```python
from build123d import *
from build123d.topology import SkipClean

# Parameters (mm, degrees)
ESBO_O1_W                = 2
ESBO_O1_H                = 46
RESSALTO_EXTRUS_O1_DEPTH = 10
ESBO_O2_W                = 46
ESBO_O2_H                = 46
RESSALTO_EXTRUS_O2_DEPTH = 3
ESBO_O1_4_W              = 2
ESBO_O1_4_H              = 46
RESSALTO_EXTRUS_O3_DEPTH = 11
ESBO_O3_R                = 11
CORTE_EXTRUS_O1_DEPTH    = 11


with BuildPart() as part:
    # Esbo_o1 → Ressalto-extrus_o1 (new body)
    with BuildSketch(Plane(origin=(0, 0, 0), x_dir=(1, 0, 0), z_dir=(0, 1, 0))):
        Polygon((0, -23), (0, -21), (-19, -21), (-19, 21), (19, 21), (19, 0), (19, -21), (5, -21), (5, -23), (7, -23), (21, -23), (21, 23), (7, 23), (3.4e-08, 23), (-7, 23), (-21, 23), (-21, -23), (-7, -23), align=None)
        Polygon((5, -21), (0, -21), (0, -23), (4.898979486, -23), (5, -23), align=None)
        with Locations((-22, 0)):
            Rectangle(ESBO_O1_W, ESBO_O1_H)
        with Locations((22, 0)):
            Rectangle(ESBO_O1_W, ESBO_O1_H)
    extrude(amount=RESSALTO_EXTRUS_O1_DEPTH)

    # Esbo_o2 → Ressalto-extrus_o2 (add)
    # profile 1 of 2: a face of its own
    with BuildSketch(Plane(origin=(0, 10, 0), x_dir=(1, 0, 0), z_dir=(0, 1, 0))):
        Rectangle(ESBO_O2_W, ESBO_O2_H)
        Polygon((19, 21), (19, 11), (19, -11), (19, -21), (-19, -21), (-19, 21), align=None, mode=Mode.SUBTRACT)
    # profile 2 of 2: a face of its own
    with BuildSketch(Plane(origin=(0, 10, 0), x_dir=(1, 0, 0), z_dir=(0, 1, 0))):
        Polygon((-9, -11), (-9, 11), (9, 11), (19, 11), (19, 21), (-19, 21), (-19, -21), (19, -21), (19, -11), (9, -11), align=None)
    extrude(amount=RESSALTO_EXTRUS_O2_DEPTH)

    # Esbo_o1_4 → Ressalto-extrus_o3 (add)
    # profile 1 of 6: a face of its own
    with SkipClean():  # the faces are left unmerged after this step: merging them gives an invalid solid
        with BuildSketch(Plane(origin=(0, 0, 0), x_dir=(1, 0, 0), z_dir=(0, 1, 0))):
            Polygon((0, -23), (0, -21), (-19, -21), (-19, 21), (19, 21), (19, 0), (19, -21), (5, -21), (5, -23), (7, -23), (21, -23), (21, 23), (7, 23), (3.4e-08, 23), (-7, 23), (-21, 23), (-21, -23), (-7, -23), align=None)
        # profile 2 of 6: a face of its own
        with BuildSketch(Plane(origin=(0, 0, 0), x_dir=(1, 0, 0), z_dir=(0, 1, 0))):
            with BuildLine():
                Line((4.898979486, -23), (0, -23))
                Line((0, -23), (-7, -23))
                Line((-7, -23), (-7, -28))
                ThreePointArc((-7, -28), (0, -35), (7, -28))
                Line((7, -28), (7, -23))
                Line((7, -23), (5, -23))
                Line((5, -23), (5, -23.101020514))
                ThreePointArc((5, -23.101020514), (4.949747468, -23.050252532), (4.898979486, -23))
            make_face()
            with BuildLine():
                ThreePointArc((5, -28), (-3.535533906, -31.535533906), (0, -23))
                ThreePointArc((0, -23), (3.535533906, -24.464466094), (5, -28))
            make_face(mode=Mode.SUBTRACT)
        # profile 3 of 6: a face of its own
        with BuildSketch(Plane(origin=(0, 0, 0), x_dir=(1, 0, 0), z_dir=(0, 1, 0))):
            Polygon((5, -21), (0, -21), (0, -23), (4.898979486, -23), (5, -23), align=None)
        # profile 4 of 6: a face of its own
        with BuildSketch(Plane(origin=(0, 0, 0), x_dir=(1, 0, 0), z_dir=(0, 1, 0))):
            with Locations((22, 0)):
                Rectangle(ESBO_O1_4_W, ESBO_O1_4_H)
        # profile 5 of 6: a face of its own
        with BuildSketch(Plane(origin=(0, 0, 0), x_dir=(1, 0, 0), z_dir=(0, 1, 0))):
            with BuildLine():
                Line((-7, 28), (-7, 23))
                Line((-7, 23), (3.4e-08, 23))
                Line((3.4e-08, 23), (7, 23))
                Line((7, 23), (7, 28))
                ThreePointArc((7, 28), (0, 35), (-7, 28))
            make_face()
            with BuildLine():
                ThreePointArc((5, 28), (3.535533918, 24.464466106), (3.4e-08, 23))
                ThreePointArc((3.4e-08, 23), (-3.535533918, 31.535533894), (5, 28))
            make_face(mode=Mode.SUBTRACT)
        # profile 6 of 6: a face of its own
        with BuildSketch(Plane(origin=(0, 0, 0), x_dir=(1, 0, 0), z_dir=(0, 1, 0))):
            with Locations((-22, 0)):
                Rectangle(ESBO_O1_4_W, ESBO_O1_4_H)
        extrude(amount=-RESSALTO_EXTRUS_O3_DEPTH)

    # Esbo_o3 → Corte-extrus_o1 (cut)
    with BuildSketch(Plane.ZY.offset(23)):
        with Locations((0, -11)):
            Circle(ESBO_O3_R)
    extrude(amount=-CORTE_EXTRUS_O1_DEPTH, mode=Mode.SUBTRACT)


solid = part.part
```
Could you check a few things on this model? Use its own coordinates, in mm. A direction names the side the tool comes from. Coordinates: 2 decimals unless noted, no trailing zeros. Order: outer loops, then holes, each group sorted by start corner. A loop starts at its lowest first (then second) coordinate and runs counter-clockwise, first axis right, second up. Notation, with made-up numbers: M -22.75,-28.5 L -4.75,-28.5 A15 cw -4.75,-16.5 Z; hole C 16.5,76 d1. An arc over 180 degrees is marked long. Use one line per item in the form item = value. Start each with the question number.
1. For pin 1 (3 mm diameter, centred on x = 14.5, z = 25.5, fed in from +Y); pin 2 (6.5 mm diameter, centred on x = 6, y = -5, fed in from -Z); pin 3 (2.5 mm diameter, centred on x = 10.5, y = 11.5, fed in from -Z); pin 4 (6 mm diameter, centred on x = 2, z = -29.5, fed in from +Y), each with a flat end and sliding along its axis, tell me the tip position at first contact or that it passes through.
2. Suppose I cut it at B-B on x = -3.5. Write out the boundary of the cut face in (y, z).
3. On a 3-axis mill with a long thin cutter (end or side, diameter ignored), from which of +Z, -Z, +X, -X, +Y, -Y can I reach the whole of each face in a straight line? I mean faces 1 (the flat face through (7, -5, -25)), 2 (the flat face through (-19, 2, 0)), 3 (the flat face through (-7, -5, -26)), 4 (the flat face through (5, 11, -11)), 5 (the flat face through (-7, -5, 25)). Say none if no direction works.
4. Suppose I cut it at D-D on z = 12.5. Write out the boundary of the cut face in (x, y).
5. Suppose I cut it at C-C on y = 6.75. Write out the boundary of the cut face in (x, z), then the cut area to 3 significant figures.
6. Please list where these lines run through material, in increasing order: line 1 (X direction, y = -1, z = -17.5); line 2 (Z direction, x = -15.5, y = -4.75); line 3 (X direction, y = -7, z = 28).
7. Suppose I cut it at A-A on z = 0. Write out the boundary of the cut face in (x, y), then the cut area to 3 significant figures.
Geometry says:
q1.pin_1 = through
q1.pin_2 = -34.44
q1.pin_3 = -23
q1.pin_4 = 0
q2.outline = M -11,-34.06 L 0,-34.06 L 0,-31.57 L -11,-31.57 Z; M -11,-24.43 L 0,-24.43 L 0,-23 L 13,-23 L 13,-11 L 10,-11 L 10,-21 L -11,-21 Z; M -11,21 L 10,21 L 10,11 L 13,11 L 13,23 L 0,23 L 0,24.43 L -11,24.43 Z; M -11,31.57 L 0,31.57 L 0,34.06 L -11,34.06 Z
q3.face_1 = -Z, +X, +Y, -Y
q3.face_2 = -Y
q3.face_3 = -Z, -X, +Y, -Y
q3.face_4 = +Y, -Y
q3.face_5 = +Z, -X, +Y, -Y
q4.outline = M -23,-11 L -19,-11 L -19,10 L 19,10 L 19,-11 L 23,-11 L 23,13 L -23,13 Z
q5.outline = M -23,-23 L 23,-23 L 23,23 L -23,23 Z; hole M -19,-21 L 19,-21 L 19,21 L -19,21 Z
q5.area = 520 mm^2
q6.line_1 = -23 to -19, 19 to 23
q6.line_2 = -23 to -21, 21 to 23
q6.line_3 = -7 to -5, 5 to 7
q7.outline = M -23,0 L -19,0 L -19,10 L -9,10 L -9,13 L -23,13 Z; M 19,-11 L 23,-11 L 23,13 L 19,13 Z
q7.area = 178 mm^2
